```python
from build123d import *

# Parameters (mm, degrees)
SKETCH1_W           = 41.148
SKETCH1_H           = 12.7
BOSS_EXTRUDE1_DEPTH = 9.525
SKETCH1_3_W         = 3.048
SKETCH1_3_H         = 7.62
BOSS_EXTRUDE2_DEPTH = 6.2865
SKETCH4_R           = 1.5
CUT_EXTRUDE3_DEPTH  = 13.7
SKETCH5_R           = 3.81
SKETCH5_R_2         = 1.5
CUT_EXTRUDE4_DEPTH  = 6.35


with BuildPart() as part:
    # Sketch1 → Boss-Extrude1 (new body, symmetric)
    with BuildSketch(Plane(origin=(0, 0, 0), x_dir=(0, 0, -1), z_dir=(1, 0, 0))):
        with Locations((0, 6.35)):
            Rectangle(SKETCH1_W, SKETCH1_H)
    extrude(amount=BOSS_EXTRUDE1_DEPTH, both=True)

    # Sketch1_3 → Boss-Extrude2 (add, symmetric)
    with BuildSketch(Plane(origin=(0, 0, 0), x_dir=(0, 0, -1), z_dir=(1, 0, 0))):
        with Locations((0, 16.51)):
            Rectangle(SKETCH1_3_W, SKETCH1_3_H)
    extrude(amount=BOSS_EXTRUDE2_DEPTH, both=True)

    # Sketch4 → Cut-Extrude3 (cut, through all)
    with BuildSketch(Plane(origin=(0, 12.7, 0), x_dir=(1, 0, 0), z_dir=(0, 1, 0))):
        with Locations((0, -14.224)):
            Circle(SKETCH4_R)
        with Locations((0, 14.224)):
            Circle(SKETCH4_R)
    extrude(amount=-CUT_EXTRUDE3_DEPTH, mode=Mode.SUBTRACT)

    # Sketch5 → Cut-Extrude4 (cut)
    with BuildSketch(Plane.XZ):
        with BuildLine():
            Line((-9.525, -18.034), (1.6e-08, -18.034))
            ThreePointArc((1.6e-08, -18.034), (-3.81, -14.224000002), (1.3e-08, -10.414))
            Line((1.3e-08, -10.414), (-9.525, -10.414))
            Line((-9.525, -10.414), (-9.525, -18.034))
        make_face()
        with Locations((0, -14.224)):
            Circle(SKETCH5_R)
        with Locations((0, -14.224)):
            Circle(SKETCH5_R_2, mode=Mode.SUBTRACT)
        with BuildLine():
            Line((1.6e-08, -18.034), (9.525, -18.034))
            Line((9.525, -18.034), (9.525, -10.414))
            Line((9.525, -10.414), (1.3e-08, -10.414))
            ThreePointArc((1.3e-08, -10.414), (2.694076841, -11.529923168), (3.81, -14.224))
            ThreePointArc((3.81, -14.224), (2.694076842, -16.91807683), (1.6e-08, -18.034))
        make_face()
        with BuildLine():
            Line((1.2e-08, 10.414), (9.525, 10.414))
            Line((9.525, 10.414), (9.525, 18.034))
            Line((9.525, 18.034), (0, 18.034))
            ThreePointArc((0, 18.034), (2.694076836, 16.918076836), (3.81, 14.224))
            ThreePointArc((3.81, 14.224), (2.694076841, 11.529923168), (1.2e-08, 10.414))
        make_face()
        with Locations((0, 14.224)):
            Circle(SKETCH5_R)
        with Locations((0, 14.224)):
            Circle(SKETCH5_R_2, mode=Mode.SUBTRACT)
        with BuildLine():
            Line((-9.525, 10.414), (1.2e-08, 10.414))
            ThreePointArc((1.2e-08, 10.414), (-3.81, 14.223999994), (0, 18.034))
            Line((0, 18.034), (-9.525, 18.034))
            Line((-9.525, 18.034), (-9.525, 10.414))
        make_face()
    extrude(amount=-CUT_EXTRUDE4_DEPTH, mode=Mode.SUBTRACT)


solid = part.part
```
Design review of the part built by this model. Coordinates are the model's own, in mm. A direction names the side the tool comes from. Coordinates: 2 decimals unless noted, no trailing zeros. Order: outer loops, then holes, each group sorted by start corner. A loop starts at its lowest first (then second) coordinate and runs counter-clockwise, first axis right, second up. Notation, with made-up numbers: (80.5, 53) -> (94.5, 53) arc R33 cw to (94.5, 88) -> close; hole circle Ø11 at (-26.75, 2.5). An arc over 180 degrees is marked (long way). One line per item, written item: value. Start each with the question number.
Q1. Take a section at D-D, the plane z = -11. State the section outline as (x, y) points (3 decimals), then the cut area to 3 significant figures.
Q2. Tool access review of faces 1 (the flat face through (-6.286, 17, 0)), 2 (the flat face through (0, 16, -1.524)), 3 (the flat face through (0, 3, -18.034)), 4 (the flat face through (0, 16, 1.524)), 5 (the flat face through (6.286, 17, 0)): name each direction out of +Z, -Z, +X, -X, +Y, -Y from which nothing blocks a thin tool from reaching the whole face with its end or side.
Q3. Take a section at C-C, the plane x = 7. State the section outline as (y, z) points, then the cut area to 3 significant figures.
Q4. Take a section at B-B, the plane x = 0. State the section outline as (y, z) points.
Q5. Mouldability with a two-part tool opening along Z and no side actions: class faces 6 (the flat face through (0, 6, -20.574)), 7 (the flat face through (0, 3, -10.414)), 8 (the flat face through (-9.525, 6, 0)) as pulls with the +Z half, pulls with the -Z half, needs draft (parallel to the pull), parting line crosses it, or undercut.
Q6. For probe 1 along Z at (x, y) = (-3.25, 5.25); probe 2 along Z at (x, y) = (0, 9); probe 3 along Y at (x, z) = (-8.5, 4), list the stretches that pass through material, from the lowest coordinate up.
Q7. Insertion check: pin 1 Ø2.5 at (x, y) = (-1.5, 18) entering from -Z; pin 2 Ø4 at (x, z) = (5.5, 16) entering from +Y; pin 3 Ø4 at (x, z) = (2, -14.5) entering from -Y; pin 4 Ø1.5 at (y, z) = (16.5, 3) entering from +X. Each pin has a flat end and moves straight along its axis. Give the tip position at first contact, or say it passes through.
Q8. Take a section at A-A, the plane y = 5.5. State the section outline as (x, z) points (3 decimals).
Values follow:
1. outline: (-9.525, 6.35) -> (9.525, 6.35) -> (9.525, 12.7) -> (-9.525, 12.7) -> close
1. area: 121 mm2
2. face 1: +Z, -Z, -X, +Y
2. face 2: -Z, +X, -X, +Y
2. face 3: +X, -X, -Y
2. face 4: +Z, +X, -X, +Y
2. face 5: +Z, -Z, +X, +Y
3. outline: (0, -20.57) -> (12.7, -20.57) -> (12.7, 20.57) -> (0, 20.57) -> (0, 18.03) -> (6.35, 18.03) -> (6.35, 10.41) -> (0, 10.41) -> (0, -10.41) -> (6.35, -10.41) -> (6.35, -18.03) -> (0, -18.03) -> close
3. area: 426 mm2
4. outline: (0, -20.57) -> (12.7, -20.57) -> (12.7, -15.72) -> (6.35, -15.72) -> (6.35, -18.03) -> (0, -18.03) -> close; (0, -10.41) -> (6.35, -10.41) -> (6.35, -12.72) -> (12.7, -12.72) -> (12.7, -1.52) -> (20.32, -1.52) -> (20.32, 1.52) -> (12.7, 1.52) -> (12.7, 12.72) -> (6.35, 12.72) -> (6.35, 10.41) -> (0, 10.41) -> close; (0, 18.03) -> (6.35, 18.03) -> (6.35, 15.72) -> (12.7, 15.72) -> (12.7, 20.57) -> (0, 20.57) -> close
5. face 6: pulls with the -Z half
5. face 7: undercut
5. face 8: needs draft
6. probe 1: z = -20.57 to -18.03, -10.41 to 10.41, 18.03 to 20.57
6. probe 2: z = -20.57 to -15.72, -12.72 to 12.72, 15.72 to 20.57
6. probe 3: y = 0 to 12.7
7. pin 1: stops at z = -1.52
7. pin 2: stops at y = 12.7
7. pin 3: stops at y = 6.35
7. pin 4: passes through
8. outline: (-9.525, -20.574) -> (9.525, -20.574) -> (9.525, -18.034) -> (-9.525, -18.034) -> close; (-9.525, -10.414) -> (9.525, -10.414) -> (9.525, 10.414) -> (-9.525, 10.414) -> close; (-9.525, 18.034) -> (9.525, 18.034) -> (9.525, 20.574) -> (-9.525, 20.574) -> close
